Autodesk Inventor part; units mm, degrees
ref_plane "Work Plane1" through (29, 0, 0) normal (0, -1, 0) x (1, 0, 0)
ref_plane "YZ Plane" through (0, 0, 0) normal (1, 0, 0) x (0, 1, 0)
ref_plane "XZ Plane" through (0, 0, 0) normal (0, 1, 0) x (-1, 0, 0)
sketch "Rascunho1" plane through (0, 0, 0) normal (0, 0, 1) x (1, 0, 0)
  line L0 (-2.3333, 0) -> (40, 0)
  line L1 (40, 0) -> (40, 5)
  line L2 (40, 5) -> (3.75, 5)
  line L3 (3.75, 5) -> (2.8297, 5)
  line L4 (2.8297, 5) -> (0, 5)
  line L5 (0, 5) -> (0, 8)
  line L6 (0, 8) -> (-10, 8)
  line L7 (-10, 8) -> (-10, 4.6188)
  line L8 (-10, 4.6188) -> (-5, 4.6188)
  line L9 (-5, 4.6188) -> (-2.3333, 0)
  line L10 (-20, 0) -> (50, 0)
  line L11 (0, -1.6) -> (0, 9.6)
  line L12 (3.75, 5) -> (0, 5) construction
  dimension "d1" = 36.25
  dimension "d2" = 0.9203
  dimension "d3" = 10
  dimension "d4" = 5
  dimension "d5" = 60
  dimension "d6" = 10
  dimension "d7" = 10
  dimension "d8" = 9.2376
  dimension "d9" = 16
  dimension "d26" = 40
revolve "Corpo" add sketch "Rascunho1" angle 360 about axis through (-2.3333, 0, 0) along (1, 0, 0)
sketch "Rascunho2" plane through (-10, 0, 0) normal (-1, 0, 0) x (0, 0, 1)
  circle A0 centre (0, 0) radius 4.6188
  line L0 (0, -11.2) -> (0, 11.2)
  line L1 (-11.2, 0) -> (11.2, 0)
  line L2 (4.6188, 0) -> (2.3094, -4)
  line L3 (2.3094, -4) -> (-2.3094, -4)
  line L4 (-2.3094, -4) -> (-4.6188, 0)
  line L5 (-4.6188, 0) -> (-2.3094, 4)
  line L6 (-2.3094, 4) -> (2.3094, 4)
  line L7 (2.3094, 4) -> (4.6188, 0)
extrude "Fenda" add sketch "Rascunho2" against normal up to next contours L7 A0 | A0 L2 | L6 L0 A0 | A0 L0 L3 | L0 L6 A0 | A0 L3 L0 | L4 A0 | A0 L5
fillet "Raio de arredondamento1" radius 1 1 edges at (-10, -8, 0)
thread "Rosca"
chamfer "Chanfrar1" distance 0.9202 distance2 0.9202 1 edges at (40, -5, 0) measured on face at (40, -1.105, 0.7295)
ref_plane "Work Plane1" through (29, 0, 0) normal (0, -1, 0) x (1, 0, 0)
fillet "Fillet2" radius 0.1 1 edges at (0, -5, 0)
equation "\"d1\" = GEL"
equation "\"d3\" = KOH"
equation "\"d4\" = INTI"
equation "\"d6\" = GD"
equation "\"d7\" = BDM"
equation "\"d8\" = 1.1547 * SW"
equation "\"d9\" = KOD"
equation "\"d26\" = NLG"
equation "\"d17\" = RR"
equation "\"d13\" = GEL"
equation "\"d15\" = -0.5 * SPD + 0.5 * GD"
equation "\"d16\" = GUL"
equation "\"d30\" = R"
equation "\"GD\" = NND"
equation "\"NLG\" = 40"
equation "\"GEL\" = 36.25"
equation "\"KOD\" = 16"
equation "\"KOH\" = 10"
equation "\"INTI\" = 5"
equation "\"GAL\" = 0.61345 * PTC"
equation "\"GUL\" = 0.61345 * PTC"
equation "\"BDM\" = NND"
equation "\"SW\" = 8"
equation "\"RR\" = 0.1 * KOH"
equation "\"SPD\" = NND - 1.2269 * PTC"
equation "\"R\" = 0.1"
equation "\"TOA\" = 30deg"
equation "\"GD1\" = THREADDIA - 1.2269 * PTC"
equation "\"FAWI\" = 45deg"
equation "\"ANG\" = 120deg"
equation "\"PTC\" = 1.5"
equation "\"E0\" = 1.155 * SW"
properties part number "DIN 912 - M10 x 40 (c)" material "Aço Inox AISI 304"
The model under review builds one solid part; all positions refer to its coordinate system, in mm. A direction names the side the tool comes from. Coordinates: 2 decimals unless noted, no trailing zeros. Loops run counter-clockwise (first coordinate to the right, second up) from the corner with the lowest first, then second, coordinate; pieces in that order, holes last. Notation, with made-up numbers: (17, -18) -> (60, -18) arc R4 ccw to (60, -13) -> close; hole circle Ø6 at (-24.5, 6.25). An arc over 180 degrees is marked (long way). Use a Markdown table: item, result. Add a question column.
1. Draft analysis for pull direction Z (two halves, no side actions). For faces 1 (the face through (-7.359, 2.028, 3.448)), 2 (the face through (-4.56, -1.73, 7.81)), 3 (the face through (0, 5, -2)), 4 (the face through (-7, -4, 0)), state which applies: pulls with the +Z half, pulls with the -Z half, needs draft (parallel to the pull), parting line crosses it, or undercut.
2. Add section A-A on x = 35. Write out the cut boundary in (y, z), plus the area to 3 significant figures.
3. To check wall thickness, follow line 1 (X direction, y = -0.5, z = 6); line 2 (Y direction, x = 34, z = 3). State the ranges of each line that lie inside material, in increasing order.
4. Machinability: for faces 5 (the face through (19.32, -1.08, 4.88)), 6 (the face through (-10, -5, 0)), 7 (the face through (-7, 4, 0)), which of the approach directions +Z, -Z, +X, -X, +Y, -Y give a long, thin tool a straight path to every point of the face, cutting with its end or side? Answer none if there is none.
5. Clearance check with flat-ended pins moving along their axes: pin 1 Ø6 at (x, y) = (20.5, 5.5) entering from +Z; pin 2 Ø4 at (x, y) = (27.5, 0) entering from +Z; pin 3 Ø2 at (x, y) = (-2.5, 6) entering from +Z (3 decimals). State where each tip first meets the part, or that it passes through.
Returned:
| question | item | result |
|---|---|---|
| 1 | face 1 | undercut |
| 1 | face 2 | parting line crosses it |
| 1 | face 3 | needs draft |
| 1 | face 4 | undercut |
| 2 | outline | circle Ø10 at (0, 0) |
| 2 | area | 78.5 mm² |
| 3 | line 1 | x = -10 to 0 |
| 3 | line 2 | y = -4 to 4 |
| 4 | face 5 | +X |
| 4 | face 6 | +Z, -Z, -X, +Y, -Y |
| 4 | face 7 | -X |
| 5 | pin 1 | stops at z = 4.33 |
| 5 | pin 2 | stops at z = 5 |
| 5 | pin 3 | stops at z = 6.245 |
